Job drawing, mm, ordinate dimensions from the low corner. One solid piece. Coordinates: 2 decimals unless noted, no trailing zeros. Write each loop counter-clockwise with the first axis right and the second up, starting at its lowest first coordinate (ties: lowest second). Pieces come first, ordered by that corner, then holes. Notation, with made-up numbers: (18, -20) -> (35, -20) arc R10 ccw to (35, -8) -> close; hole circle Ø9 at (49, -31.5). An arc over 180 degrees is marked (long way). Answer as a JSON object with one key per item and string values. Group by question number.
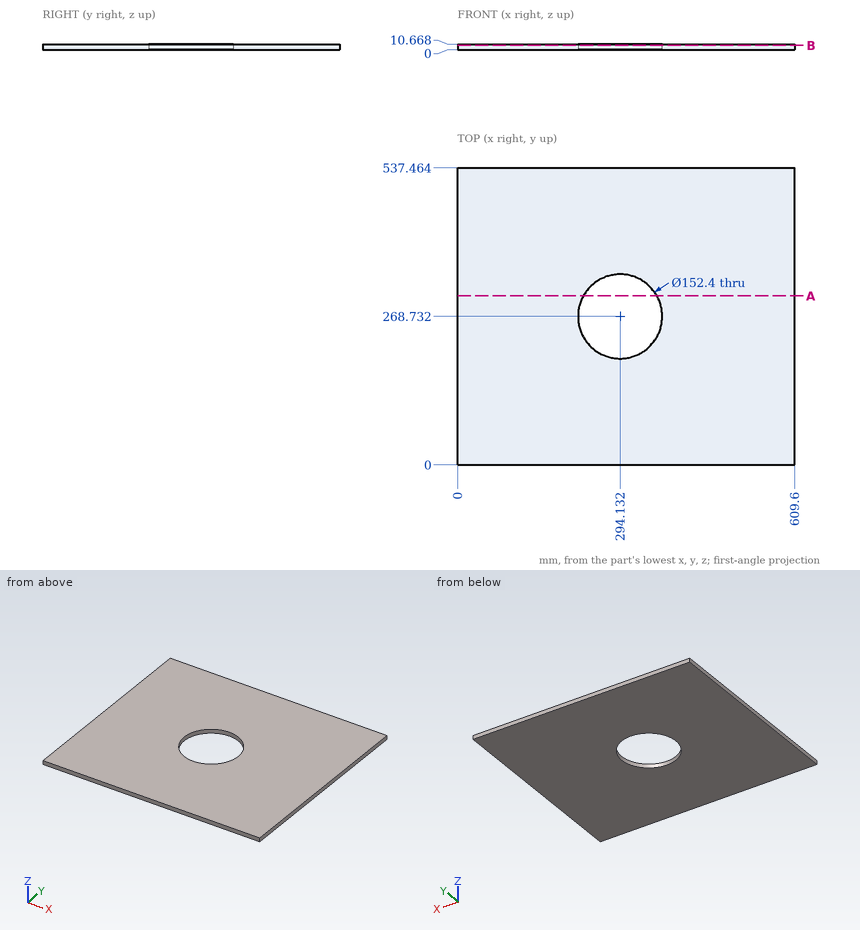
(1) Wall check: probe 1 along Y at (x, z) = (270, 5.75); probe 2 along Y at (x, z) = (271.5, 6); probe 3 along X at (y, z) = (246, 8.25). Give the ranges that are in metal, low to high.
(2) Cut at A-A on y = 306. List the corners of the cut face in (x, z).
(3) Cut at B-B on z = 8. List the corners of the cut face in (x, y), plus the area to 3 significant figures.
Results found:
{
 "1": {"probe 1": "y = 0 to 196.45, 341.01 to 537.46", "probe 2": "y = 0 to 195.97, 341.49 to 537.46", "probe 3": "x = 0 to 221.4, 366.86 to 609.6"},
 "2": {"outline": "(0, 0) -> (227.67, 0) -> (227.67, 10.67) -> (0, 10.67) -> close; (360.6, 0) -> (609.6, 0) -> (609.6, 10.67) -> (360.6, 10.67) -> close"},
 "3": {"outline": "(0, 0) -> (609.6, 0) -> (609.6, 537.46) -> (0, 537.46) -> close; hole circle Ø152.4 at (294.13, 268.73)", "area": "309,000 mm²"}
}
